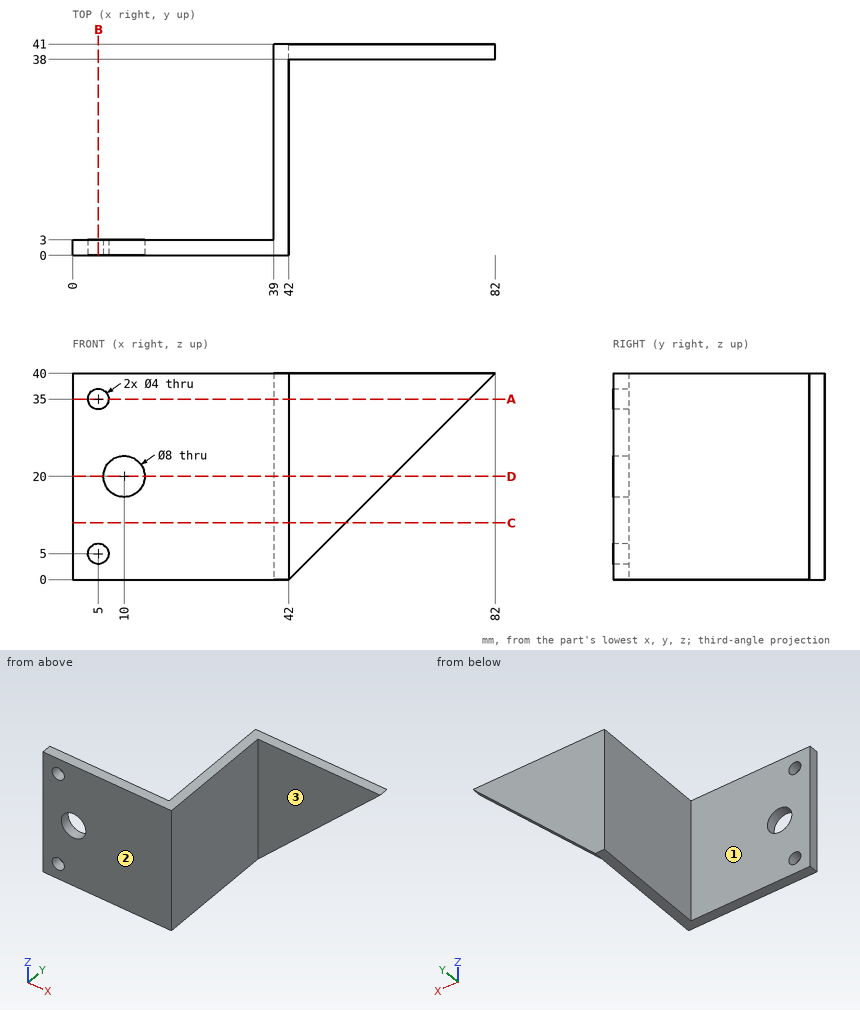
Input: dimensioned drawing with shaded views. Units: mm. Origin: part minimum x, y, z. A direction names the side the tool comes from. Coordinates: 2 decimals unless noted, no trailing zeros. Loops run counter-clockwise (first coordinate to the right, second up) from the corner with the lowest first, then second, coordinate; pieces in that order, holes last. Notation, with made-up numbers: M 70,45 L 90,45 A32 cw 90,82 Z; hole C 24,49.25 d1. An arc over 180 degrees is marked long. Use a Markdown table: item, result. Add a question column.
Q1. Section query D-D, the plane z = 20. Return loops of the section in (x, y).
Q2. Section query A-A, the plane z = 35. Return loops of the section in (x, y), and give its area (3 significant figures).
Q3. First-contact query: pin 1 (4 mm diameter, centred on y = 6, z = 13.5, fed in from -X); pin 2 (1.5 mm diameter, centred on y = 35, z = 33, fed in from +X); pin 3 (20 mm diameter, centred on x = 54, z = 27.5, fed in from -Y). Flat tips, straight axial feed; report the tip coordinate or a pass-through.
Q4. Material intervals for L1, parallel to X at y = 0.7, z = 20; L2, parallel to Y at x = 17.5, z = 28; L3, parallel to X at y = 19.5, z = 30, sorted ascending.
Q5. Section query C-C, the plane z = 11. Return loops of the section in (x, y), and give its area (3 significant figures).
Q6. Access query for the marked faces 1, 2 and 3. Directions: +Z, -Z, +X, -X, +Y, -Y. A direction counts if a zero-diameter tool reaches every point of the face in a straight line with its end or side. Return the directions, or none.
Q7. Section query B-B, the plane x = 5. Return loops of the section in (y, z), and give its area (3 significant figures).
Result:
| question | item | result |
|---|---|---|
| 1 | outline | M 0,0 L 6,0 L 6,3 L 0,3 Z; M 14,0 L 42,0 L 42,38 L 62,38 L 62,41 L 39,41 L 39,3 L 14,3 Z |
| 2 | outline | M 0,0 L 3,0 L 3,3 L 0,3 Z; M 7,0 L 42,0 L 42,38 L 77,38 L 77,41 L 39,41 L 39,3 L 7,3 Z |
| 2 | area | 333 mm2 |
| 3 | pin 1 | stops at x = 39 |
| 3 | pin 2 | stops at x = 42 |
| 3 | pin 3 | stops at y = 38 |
| 4 | L1 | x = 0 to 6, 14 to 42 |
| 4 | L2 | y = 0 to 3 |
| 4 | L3 | x = 39 to 42 |
| 5 | outline | M 0,0 L 42,0 L 42,38 L 53,38 L 53,41 L 39,41 L 39,3 L 0,3 Z |
| 5 | area | 273 mm2 |
| 6 | face 1 | +Z, -Z, -X, +Y |
| 6 | face 2 | +Z, -Z, +X, -X, -Y |
| 6 | face 3 | +Z, -Z, +X, -Y |
| 7 | outline | M 0,0 L 3,0 L 3,3 L 0,3 Z; M 0,7 L 3,7 L 3,33 L 0,33 Z; M 0,37 L 3,37 L 3,40 L 0,40 Z |
| 7 | area | 96.0 mm2 |
